Read the model definition and answer for the solid it produces. Units are mm, in the model's axes. A direction names the side the tool comes from. Coordinates: 2 decimals unless noted, no trailing zeros. Order: outer loops, then holes, each group sorted by start corner. A loop starts at its lowest first (then second) coordinate and runs counter-clockwise, first axis right, second up. Notation, with made-up numbers: (-8.5, -10) - (35.5, -10) arc R31 ccw to (35.5, 28) - close; hole circle Ø3 at (64.25, -15). An arc over 180 degrees is marked (long way). Answer as a JSON object with one key per item and string values. Group by question number.
from build123d import *

# Parameters (mm, degrees)
F1_DEPTH = 63.5
F0_W     = 25.4
F0_H     = 19.05
F2_DEPTH = 25.4
F3_DEPTH = 8.255


with BuildPart() as f1:
    # F0 (on Front) → F1 (new body, symmetric)
    with BuildSketch(Plane.XZ):
        Polygon((41.275, -9.525), (41.275, 9.525), (22.225, 9.525), (-41.275, 9.525), (-41.275, -9.525), align=None)
    extrude(amount=F1_DEPTH, both=True)

    # F0 (on Front) → F2 (join, symmetric)
    with BuildSketch(Plane.XZ):
        with BuildLine():
            Line((22.225, 9.525), (41.275, 9.525))
            Line((41.275, 9.525), (41.275, 27.0002))
            ThreePointArc((41.275, 27.0002), (45.9246798487, 38.2255201513), (57.15, 42.8752))
            Line((57.15, 42.8752), (60.325, 42.8752))
            Line((60.325, 42.8752), (60.325, 61.9252))
            Line((60.325, 61.9252), (57.15, 61.9252))
            ThreePointArc((57.15, 61.9252), (32.4542956671, 51.6959043329), (22.225, 27.0002))
            Line((22.225, 27.0002), (22.225, 9.525))
        make_face()
        with Locations((73.025, 52.4002)):
            Rectangle(F0_W, F0_H)
    extrude(amount=F2_DEPTH, both=True)

    # F0 (on Front) → F3 (join, symmetric)
    with BuildSketch(Plane.XZ):
        with BuildLine():
            Line((-41.275, 9.525), (22.225, 9.525))
            Line((22.225, 9.525), (22.225, 27.0002))
            ThreePointArc((22.225, 27.0002), (32.4542956671, 51.6959043329), (57.15, 61.9252))
            add(Edge.make_bspline(
                [(-41.275, 9.525), (-41.275, 38.1), (16.719141975, 61.9252), (57.15, 61.9252)],
                knots=[0, 0, 0, 0, 111.5045361635, 111.5045361635, 111.5045361635, 111.5045361635], degree=3))
        make_face()
    extrude(amount=F3_DEPTH, both=True)

    # F0 (on Front) → F4 (revolve)
    with BuildSketch(Plane.XZ):
        Polygon((85.725, 61.9252), (85.725, 42.8752), (85.725, 38.1), (111.125, 38.1), (111.125, 66.675), (85.725, 66.675), align=None)
    revolve(axis=Axis((85.725, 0, 52.3875), (0, 0, 1)))


solid = f1.part
1. A cutting plane is placed at A-A on y = 44. Write down the section's boundary in (x, z) (3 decimals), and give its area (3 significant figures).
2. Given pin 1 (15 mm diameter, centred on x = 97.5, y = 5.5, fed in from -Z); pin 2 (16.5 mm diameter, centred on x = 18.5, y = -22.5, fed in from +Z); pin 3 (15.5 mm diameter, centred on x = 15.5, z = 27.5, fed in from +Y), each flat-ended and moving along its own axis, determine where each tip first touches the part or whether it passes through.
3. For faces 1 (the flat face through (22.225, -17, 18)), 2 (the flat face through (46, 25.4, 42)), 3 (the flat face through (86, 0, 38.1)), 4 (the flat face through (-4, 8.255, 30)), determine the directions among +Z, -Z, +X, -X, +Y, -Y from which every point of the face is accessible in a straight line to the end or side of a thin tool.
4. For a pull along X with two mould halves and no side action, classify faces 5 (the flat face through (41.275, -1, 4)), 6 (the flat face through (46, -25.4, 42)), 7 (the cylindrical face through (45.8, -0.4, 38.1)) as pulls with the +X half, pulls with the -X half, needs draft (parallel to the pull), parting line crosses it, or undercut.
5. Straight lines are drawn through the part: L1, parallel to Y at x = 49.5, z = 56; L2, parallel to Z at x = 16, y = 43 (3 decimals); L3, parallel to Y at x = -34, z = 16 (3 decimals). For each, find the intervals that lie inside material, in ascending order.
6. A cutting plane is placed at B-B on z = 6. Write down the section's boundary in (x, y) (3 decimals).
Derived:
{
 "1": {"outline": "(-41.275, -9.525) - (41.275, -9.525) - (41.275, 9.525) - (-41.275, 9.525) - close", "area": "1,570 mm2"},
 "2": {"pin 1": "stops at z = 38.1", "pin 2": "stops at z = 44.19", "pin 3": "stops at y = 25.4"},
 "3": {"face 1": "+Z, -X, -Y", "face 2": "+Z, +X, -X, +Y", "face 3": "-Z, +X, +Y, -Y", "face 4": "+Z, -X, +Y"},
 "4": {"face 5": "pulls with the +X half", "face 6": "needs draft", "face 7": "undercut"},
 "5": {"L1": "y = -25.4 to 25.4", "L2": "z = -9.525 to 9.525", "L3": "y = -8.255 to 8.255"},
 "6": {"outline": "(-41.275, -63.5) - (41.275, -63.5) - (41.275, 63.5) - (-41.275, 63.5) - close"}
}
